Design review of the part built by this model. Coordinates are the model's own, in mm. Round coordinates to 2 decimals unless told otherwise and drop trailing zeros. Order: outer loops, then holes, each group sorted by start corner. A loop starts at its lowest first (then second) coordinate and runs counter-clockwise, first axis right, second up. Notation, with made-up numbers: M -6.75,14 L 35.25,14 A25 cw 35.25,46 Z; hole C 17,54.25 d1. An arc over 180 degrees is marked long. Write each question's results on one line, items separated by ' | '. Start each with the question number.
Item 1: Wall thickness on line 1 (X direction, y = 13, z = 1.45) (3 decimals); line 2 (X direction, y = 40.5, z = 1.6) (3 decimals); line 3 (Y direction, x = 85, z = 1.35): over which ranges is each line inside the solid? List them lowest first. Write a range as [from, to].
Item 2: Take a section at D-D, the plane x = 314.5. Write out the cut boundary in (y, z).
Item 3: Take a section at A-A, the plane y = 37.5. Write out the cut boundary in (x, z) (3 decimals).
Item 4: Take a section at C-C, the plane x = 371.5. Write out the cut boundary in (y, z).
Item 5: Clearance check with flat-ended pins moving along their axes: pin 1 (1.2 mm diameter, centred on x = 331.5, z = 1, fed in from -Y); pin 2 (1.2 mm diameter, centred on x = 231, z = 0.5, fed in from -Y); pin 3 (1 mm diameter, centred on x = 397, z = 1, fed in from -Y). State where each tip first meets the part, or that it passes through.
Item 6: Take a section at B-B, the plane z = 1.5. Write out the cut boundary in (x, y) (3 decimals), plus the area to 3 significant figures.
Autodesk Inventor part; units mm, degrees
ref_plane "YZ Plane" through (0, 0, 0) normal (1, 0, 0) x (0, 1, 0)
ref_plane "XZ Plane" through (0, 0, 0) normal (0, 1, 0) x (-1, 0, 0)
ref_plane "XY Plane" through (0, 0, 0) normal (0, 0, 1) x (1, 0, 0)
sketch "Sketch1" plane through (0, 0, 0) normal (0, 0, 1) x (1, 0, 0)
  line L0 (0, 0) -> (454.025, 0)
  line L1 (454.025, 0) -> (454.025, 127)
  line L2 (454.025, 127) -> (0, 127)
  line L3 (0, 127) -> (0, 0)
  dimension "d0" = 127
  dimension "d1" = 454.025
extrude "Extrusion1" add sketch "Sketch1" along normal blind 2.3622
sketch "Sketch2" plane through (0, 0, 2.3622) normal (0, 0, 1) x (1, 0, 0)
  line L0 (35.56, 0) -> (35.56, 8.128)
  line L1 (35.56, 8.128) -> (41.91, 8.128)
  line L2 (41.91, 8.128) -> (41.91, 18.288)
  line L3 (41.91, 18.288) -> (104.14, 18.288)
  line L4 (104.14, 18.288) -> (104.14, 8.128)
  line L5 (104.14, 8.128) -> (114.935, 8.128)
  line L6 (114.935, 8.128) -> (114.935, 18.288)
  line L7 (114.935, 18.288) -> (323.215, 18.288)
  line L8 (323.215, 18.288) -> (323.215, 8.128)
  line L9 (323.215, 8.128) -> (334.01, 8.128)
  line L10 (334.01, 8.128) -> (334.01, 48.768)
  line L11 (334.01, 48.768) -> (415.29, 48.768)
  line L12 (415.29, 48.768) -> (415.29, 8.128)
  line L13 (415.29, 8.128) -> (421.64, 8.128)
  line L14 (421.64, 8.128) -> (421.64, 0)
  line L15 (0, 127) -> (0, 0)
  line L16 (454.025, 0) -> (454.025, 127)
  line L17 (0, 0) -> (454.025, 0)
  line L18 (35.56, 0) -> (421.64, 0)
  dimension "d4" = 35.56
  dimension "d5" = 6.35
  dimension "d6" = 62.23
  dimension "d7" = 10.795
  dimension "d8" = 208.28
  dimension "d12" = 8.128
  dimension "d13" = 10.16
  dimension "d14" = 10.16
  dimension "d15" = 40.64
  dimension "d18" = 454.025
  dimension "d19" = 10.795
  dimension "d20" = 81.28
  dimension "d21" = 6.35
extrude "Extrusion2" cut sketch "Sketch2" against normal blind 2.3622
properties part number "TSIWall"
Results list:
1) line 1: [0, 41.91], [104.14, 114.935], [323.215, 334.01], [415.29, 454.025] | line 2: [0, 334.01], [415.29, 454.025] | line 3: [18.29, 127]
2) outline: M 18.29,0 L 127,0 L 127,2.36 L 18.29,2.36 Z
3) outline: M 0,0 L 334.01,0 L 334.01,2.362 L 0,2.362 Z; M 415.29,0 L 454.025,0 L 454.025,2.362 L 415.29,2.362 Z
4) outline: M 48.77,0 L 127,0 L 127,2.36 L 48.77,2.36 Z
5) pin 1: y = 8.13 | pin 2: y = 18.29 | pin 3: y = 48.77
6) outline: M 0,0 L 35.56,0 L 35.56,8.128 L 41.91,8.128 L 41.91,18.288 L 104.14,18.288 L 104.14,8.128 L 114.935,8.128 L 114.935,18.288 L 323.215,18.288 L 323.215,8.128 L 334.01,8.128 L 334.01,48.768 L 415.29,48.768 L 415.29,8.128 L 421.64,8.128 L 421.64,0 L 454.025,0 L 454.025,127 L 0,127 Z | area: 48,500 mm²
